For this review, take the finished solid that the model builds, in its own axes (mm). Face numbers are marked on the shaded views. A direction names the side the tool comes from. Round coordinates to 2 decimals unless told otherwise and drop trailing zeros. Loops run counter-clockwise (first coordinate to the right, second up) from the corner with the lowest first, then second, coordinate; pieces in that order, holes last. Notation, with made-up numbers: (32, 30) -> (53, 30) arc R4 cw to (53, 37) -> close; hole circle Ø5 at (-23, -20). An arc over 180 degrees is marked (long way). Write each question's results on one line, items separated by ' | '.
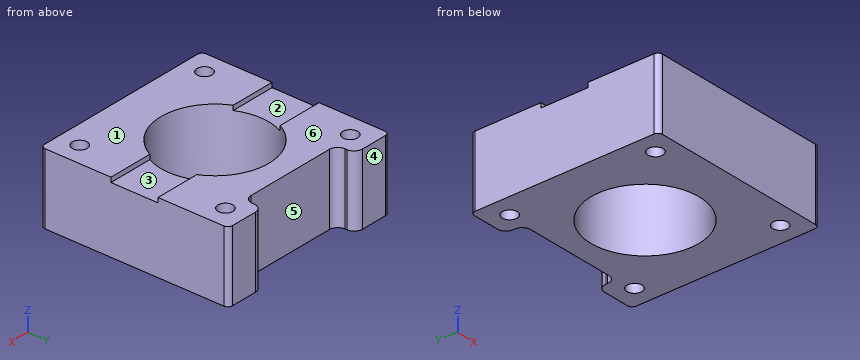
```python
from build123d import *

# Parameters (mm, degrees)
SKETCH1_R           = 11.5
SKETCH1_R_2         = 1.6
BOSS_EXTRUDE1_DEPTH = 15
SKETCH2_W           = 40
SKETCH2_H           = 10
CUT_EXTRUDE1_DEPTH  = 1


with BuildPart() as part:
    # Sketch1 → Boss-Extrude1 (new body)
    with BuildSketch(Plane.XY):
        with BuildLine():
            Line((-20, 19), (-20, -19))
            ThreePointArc((-20, -19), (-19.707106781, -19.707106781), (-19, -20))
            Line((-19, -20), (19, -20))
            ThreePointArc((19, -20), (19.707106781, -19.707106781), (20, -19))
            Line((20, -19), (20, 19))
            ThreePointArc((20, 19), (19.707106781, 19.707106781), (19, 20))
            Line((19, 20), (13.3, 20))
            ThreePointArc((13.3, 20), (12.027207794, 19.472792206), (11.5, 18.2))
            Line((11.5, 18.2), (11.5, 17.8))
            ThreePointArc((11.5, 17.8), (10.972792206, 16.527207794), (9.7, 16))
            Line((9.7, 16), (-9.7, 16))
            ThreePointArc((-9.7, 16), (-10.972792206, 16.527207794), (-11.5, 17.8))
            Line((-11.5, 17.8), (-11.5, 18.2))
            ThreePointArc((-11.5, 18.2), (-12.027207794, 19.472792206), (-13.3, 20))
            Line((-13.3, 20), (-19, 20))
            ThreePointArc((-19, 20), (-19.707106781, 19.707106781), (-20, 19))
        make_face()
        Circle(SKETCH1_R, mode=Mode.SUBTRACT)
        with Locations((-15.5, 15.5)):
            Circle(SKETCH1_R_2, mode=Mode.SUBTRACT)
        with Locations((15.5, 15.5)):
            Circle(SKETCH1_R_2, mode=Mode.SUBTRACT)
        with Locations((15.5, -15.5)):
            Circle(SKETCH1_R_2, mode=Mode.SUBTRACT)
        with Locations((-15.5, -15.5)):
            Circle(SKETCH1_R_2, mode=Mode.SUBTRACT)
    extrude(amount=BOSS_EXTRUDE1_DEPTH)

    # Sketch2 → Cut-Extrude1 (cut)
    with BuildSketch(Plane.XY.offset(15)):
        Rectangle(SKETCH2_W, SKETCH2_H)
    extrude(amount=-CUT_EXTRUDE1_DEPTH, mode=Mode.SUBTRACT)


solid = part.part
```
1. Consider section B-B (x = -15.5). State the section outline as (y, z) points, plus the area to 3 significant figures.
Values found:
outline: (-20, 0) -> (-17.1, 0) -> (-17.1, 15) -> (-20, 15) -> close; (-13.9, 0) -> (13.9, 0) -> (13.9, 15) -> (5, 15) -> (5, 14) -> (-5, 14) -> (-5, 15) -> (-13.9, 15) -> close; (17.1, 0) -> (20, 0) -> (20, 15) -> (17.1, 15) -> close | area: 494 mm2
2. To check wall thickness, follow probe 1 along Y at (x, z) = (15.5, 3.75); probe 2 along Y at (x, z) = (0.5, 3); probe 3 along X at (y, z) = (15, 12). State the ranges of each line that lie inside material, in increasing order.
Values found:
probe 1: y = -20 to -17.1, -13.9 to 13.9, 17.1 to 20 | probe 2: y = -20 to -11.49, 11.49 to 16 | probe 3: x = -20 to -17.02, -13.98 to 13.98, 17.02 to 20
3. Consider section A-A (y = 0). State the section outline as (x, z) points.
Values found:
outline: (-20, 0) -> (-11.5, 0) -> (-11.5, 14) -> (-20, 14) -> close; (11.5, 0) -> (20, 0) -> (20, 14) -> (11.5, 14) -> close
4. Draft analysis for pull direction Y (two halves, no side actions). For the marked faces 1, 2, 3 and 4, state which applies: released by +Y, released by -Y, zero draft, split by the parting line, or undercut.
Values found:
face 1: zero draft | face 2: undercut | face 3: undercut | face 4: released by +Y
5. For pin 1 (1 mm diameter, centred on x = -13.5, y = 2.5, fed in from +Z); pin 2 (4 mm diameter, centred on x = -8, z = 10, fed in from +Y), all flat-tipped, find the tip position at first contact; note any pin that passes through.
Values found:
pin 1: stops at z = 14 | pin 2: stops at y = 16.03
6. Tool access review of the marked faces 5 and 6: name each direction out of +Z, -Z, +X, -X, +Y, -Y from which nothing blocks a thin tool from reaching the whole face with its end or side.
Values found:
face 5: +Z, -Z, +Y | face 6: +Z, +X, -X, +Y, -Y
7. Consider section D-D (y = -15.5). State the section outline as (x, z) points.
Values found:
outline: (-20, 0) -> (-17.1, 0) -> (-17.1, 15) -> (-20, 15) -> close; (-13.9, 0) -> (13.9, 0) -> (13.9, 15) -> (-13.9, 15) -> close; (17.1, 0) -> (20, 0) -> (20, 15) -> (17.1, 15) -> close
8. Consider section C-C (z = 13.5). State the section outline as (x, y) points, plus the area to 3 significant figures.
Values found:
outline: (-20, -19) arc R1 ccw to (-19, -20) -> (19, -20) arc R1 ccw to (20, -19) -> (20, 19) arc R1 ccw to (19, 20) -> (13.3, 20) arc R1.8 ccw to (11.5, 18.2) -> (11.5, 17.8) arc R1.8 cw to (9.7, 16) -> (-9.7, 16) arc R1.8 cw to (-11.5, 17.8) -> (-11.5, 18.2) arc R1.8 ccw to (-13.3, 20) -> (-19, 20) arc R1 ccw to (-20, 19) -> close; hole circle Ø3.2 at (-15.5, -15.5); hole circle Ø3.2 at (-15.5, 15.5); hole circle Ø23 at (0, 0); hole circle Ø3.2 at (15.5, -15.5); hole circle Ø3.2 at (15.5, 15.5) | area: 1,060 mm2
